from build123d import *

# Parameters (mm, degrees)
SKETCH_1_W      = 30
SKETCH_1_H      = 17
EXTRUDE_1_DEPTH = 1.5
SKETCH_4_W      = 6
SKETCH_4_H      = 6
SKETCH_4_W_2    = 4.739464385
SKETCH_4_H_2    = 7.603341308
EXTRUDE_3_DEPTH = 4
SKETCH_6_W      = 5
SKETCH_6_H      = 15
SKETCH_6_W_2    = 3
EXTRUDE_4_DEPTH = 1.55


with BuildPart() as part:
    # Эскиз1 → Бобышка-Вытянуть1 (new body)
    with BuildSketch(Plane(origin=(0, 0, 0), x_dir=(1, 0, 0), z_dir=(0, 1, 0))):
        with Locations((-15, 0)):
            Rectangle(SKETCH_1_W, SKETCH_1_H)
    extrude(amount=EXTRUDE_1_DEPTH)

    # Эскиз4 → Бобышка-Вытянуть3 (add)
    with BuildSketch(Plane(origin=(0, 0, 0), x_dir=(1, 0, 0), z_dir=(0, 1, 0))):
        with Locations((-17, 4.741395497)):
            Rectangle(SKETCH_4_W, SKETCH_4_H)
        with Locations((-27.630267808, 0)):
            Rectangle(SKETCH_4_W_2, SKETCH_4_H_2)
    extrude(amount=EXTRUDE_3_DEPTH)

    # Эскиз6 → Бобышка-Вытянуть4 (add)
    with BuildSketch(Plane(origin=(0, 0, 0), x_dir=(1, 0, 0), z_dir=(0, 1, 0))):
        with Locations((-3.5, 0)):
            Rectangle(SKETCH_6_W, SKETCH_6_H)
        with Locations((-27.5, 0)):
            Rectangle(SKETCH_6_W_2, SKETCH_6_H)
    extrude(amount=EXTRUDE_4_DEPTH)


solid = part.part
The model under review builds one solid part; all positions refer to its coordinate system, in mm. A direction names the side the tool comes from. Round coordinates to 2 decimals unless told otherwise and drop trailing zeros. Loops run counter-clockwise (first coordinate to the right, second up) from the corner with the lowest first, then second, coordinate; pieces in that order, holes last. Notation, with made-up numbers: (20.25, 24) - (78.25, 24) arc R30 ccw to (78.25, 59) - close; hole circle Ø4 at (19, 59). An arc over 180 degrees is marked (long way). Use CSV: the item, a comma, the result in double quotes.
(1) Clearance check with flat-ended pins moving along their axes: P1, Ø2, axis at y = 2, z = -6, coming from the -X side; P2, Ø2, axis at x = -5, z = 6.5, coming from the +Y side; P3, Ø6, axis at x = -21, z = 3, coming from the +Y side; P4, Ø0.8, axis at x = -16, y = 2.5, coming from the -Z side. State where each tip first meets the part, or that it passes through.
Working result:
P1,"stops at x = -30"
P2,"stops at y = 1.55"
P3,"stops at y = 1.5"
P4,"stops at z = -7.74"
(2) For line 1 (X direction, y = 3.35, z = -2.25); line 2 (Y direction, x = -10, z = 1); line 3 (X direction, y = 2, z = -6), list the stretches that pass through material, from the lowest coordinate up.
Working result:
line 1,"x = -30 to -25.26, -20 to -14"
line 2,"y = 0 to 1.5"
line 3,"x = -20 to -14"
(3) Take a section at D-D, the plane z = -2.25. Give the boundary of the cut face in (x, y), plus the area to 3 significant figures.
Working result:
outline,"(-30, 0) - (0, 0) - (0, 1.5) - (-1, 1.5) - (-1, 1.55) - (-6, 1.55) - (-6, 1.5) - (-14, 1.5) - (-14, 4) - (-20, 4) - (-20, 1.5) - (-25.26, 1.5) - (-25.26, 4) - (-30, 4) - close"
area,"72.1 mm^2"
(4) Take a section at B-B, the plane z = 6. Give the boundary of the cut face in (x, y).
Working result:
outline,"(-30, 0) - (0, 0) - (0, 1.5) - (-1, 1.5) - (-1, 1.55) - (-6, 1.55) - (-6, 1.5) - (-26, 1.5) - (-26, 1.55) - (-29, 1.55) - (-29, 1.5) - (-30, 1.5) - close"
(5) Machinability: for faces 1 (the flat face through (-17, 3, -7.741)), 2 (the flat face through (-28, 1.55, 6)), 3 (the flat face through (-15, 1, 8.5)), 4 (the flat face through (-28, 1.55, -6)), 5 (the flat face through (-25.261, 3, 0)), which of the approach directions +Z, -Z, +X, -X, +Y, -Y give a long, thin tool a straight path to every point of the face, cutting with its end or side? Answer none if there is none.
Working result:
face 1,"-Z, +X, -X, +Y"
face 2,"+Z, +X, -X, +Y"
face 3,"+Z, +X, -X, +Y, -Y"
face 4,"-Z, -X, +Y"
face 5,"+Z, -Z, +Y"
(6) Take a section at C-C, the plane x = -4.5. Give the boundary of the cut face in (y, z).
Working result:
outline,"(0, -8.5) - (1.5, -8.5) - (1.5, -7.5) - (1.55, -7.5) - (1.55, 7.5) - (1.5, 7.5) - (1.5, 8.5) - (0, 8.5) - close"
(7) The part is to be moulded in two halves that separate along X. For faces 6 (the flat face through (-4, 1.55, 0)), 7 (the flat face through (-15, 1.5, 0)), 8 (the flat face through (-30, 2, 0)), 9 (the flat face through (0, 1, 0)), say which applies: pulls with the +X half, pulls with the -X half, needs draft (parallel to the pull), parting line crosses it, or undercut.
Working result:
face 6,"needs draft"
face 7,"undercut"
face 8,"pulls with the -X half"
face 9,"pulls with the +X half"
(8) Take a section at A-A, the plane y = 2. Give the boundary of the cut face in (x, z), plus the area to 3 significant figures.
Working result:
outline,"(-30, -3.8) - (-25.26, -3.8) - (-25.26, 3.8) - (-30, 3.8) - close; (-20, -7.74) - (-14, -7.74) - (-14, -1.74) - (-20, -1.74) - close"
area,"72.0 mm^2"
